Part model, mm, in its own coordinate system. Face numbers are marked on the shaded views. Round coordinates to 2 decimals unless told otherwise and drop trailing zeros. Loops run counter-clockwise (first coordinate to the right, second up) from the corner with the lowest first, then second, coordinate; pieces in that order, holes last.
from build123d import *

# Parameters (mm, degrees)
SKETCH1_W           = 40
SKETCH1_H           = 50
BOSS_EXTRUDE1_DEPTH = 5
SKETCH2_W           = 27
SKETCH2_H           = 6
SKETCH2_H_2         = 4
CUT_EXTRUDE1_DEPTH  = 6
SKETCH3_R           = 3.025
CUT_EXTRUDE2_DEPTH  = 6
LPATTERN1_COUNT     = 2
LPATTERN1_PITCH     = 12
LPATTERN1_COL_COUNT = 2
LPATTERN1_COL_PITCH = 12
FILLET1_R           = 4
FILLET2_R           = 0.5


with BuildPart() as part:
    # Sketch1 → Boss-Extrude1 (new body)
    with BuildSketch(Plane(origin=(0, 0, 0), x_dir=(1, 0, 0), z_dir=(0, 1, 0))):
        Rectangle(SKETCH1_W, SKETCH1_H)
    extrude(amount=BOSS_EXTRUDE1_DEPTH)

    # Sketch2 → Cut-Extrude1 (cut, through all)
    with BuildSketch(Plane(origin=(0, 5, 0), x_dir=(1, 0, 0), z_dir=(0, 1, 0))):
        with Locations((0, 18)):
            Rectangle(SKETCH2_W, SKETCH2_H)
        with Locations((0, 8.5)):
            Rectangle(SKETCH2_W, SKETCH2_H)
        Rectangle(SKETCH2_W, SKETCH2_H_2)
    extrude(amount=-CUT_EXTRUDE1_DEPTH, mode=Mode.SUBTRACT)

    # Sketch3 → Cut-Extrude2 (cut, through all)
    with BuildSketch(Plane(origin=(0, 5, 0), x_dir=(1, 0, 0), z_dir=(0, 1, 0))):
        with Locations((0, -10)):
            Circle(SKETCH3_R)
    cut_extrude2 = extrude(amount=-CUT_EXTRUDE2_DEPTH, mode=Mode.SUBTRACT)

    # LPattern1: Cut-Extrude2 ×2
    with Locations(*[(i * LPATTERN1_PITCH, 0, 0) for i in range(1, LPATTERN1_COUNT)]):
        add(cut_extrude2, mode=Mode.SUBTRACT)

    # LPattern1 col: Cut-Extrude2 ×2
    with Locations(*[(-i * LPATTERN1_COL_PITCH, 0, 0) for i in range(1, LPATTERN1_COL_COUNT)]):
        add(cut_extrude2, mode=Mode.SUBTRACT)

    # Fillet1
    fillet1_edges = [part.edges().sort_by_distance(p)[0] for p in [
        (20, 2.5, 25),
        (-20, 2.5, 25),
        (-20, 2.5, -25),
        (20, 2.5, -25),
    ]]
    fillet(fillet1_edges, radius=FILLET1_R)

    # Fillet2
    fillet2_edges = [part.edges().sort_by_distance(p)[0] for p in [
        (13.5, 2.5, -21),
        (13.5, 2.5, -15),
        (-13.5, 2.5, -15),
        (-13.5, 2.5, -21),
        (13.5, 2.5, -11.5),
        (13.5, 2.5, -5.5),
        (-13.5, 2.5, -5.5),
        (-13.5, 2.5, -11.5),
        (13.5, 2.5, -2),
        (13.5, 2.5, 2),
        (-13.5, 2.5, 2),
        (-13.5, 2.5, -2),
    ]]
    fillet(fillet2_edges, radius=FILLET2_R)


solid = part.part
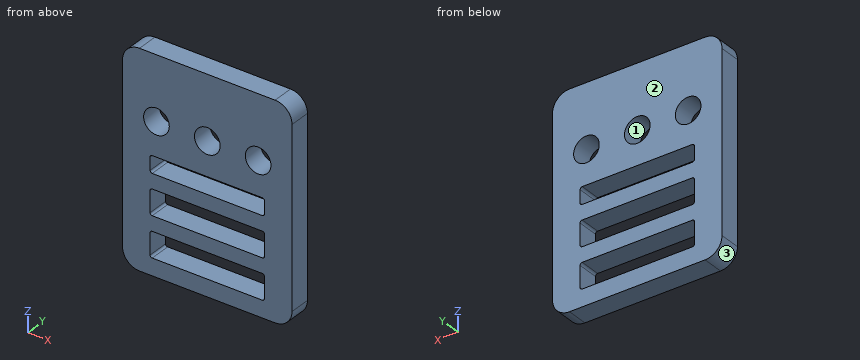
1) Slice it at A-A, the plane x = 7.5. Give the cut face in (y, z), then the cut area to 3 significant figures.
Values:
outline: (0, -25) - (5, -25) - (5, -21) - (0, -21) - close; (0, -15) - (5, -15) - (5, -11.5) - (0, -11.5) - close; (0, -5.5) - (5, -5.5) - (5, -2) - (0, -2) - close; (0, 2) - (5, 2) - (5, 25) - (0, 25) - close
area: 170 mm2
2) Slice it at B-B, the plane z = 10. Give the cut face in (x, y) (3 decimals), then the cut area to 3 significant figures.
Values:
outline: (-20, 0) - (-15.025, 0) - (-15.025, 5) - (-20, 5) - close; (-8.975, 0) - (-3.025, 0) - (-3.025, 5) - (-8.975, 5) - close; (3.025, 0) - (8.975, 0) - (8.975, 5) - (3.025, 5) - close; (15.025, 0) - (20, 0) - (20, 5) - (15.025, 5) - close
area: 109 mm2
3) Drop a flat-ended pin along its axis: pin 1 Ø3.5 at (x, z) = (12, 10) entering from -Y. Give the stop position or say it passes through.
Values:
pin 1: passes through
4) Wall check: line 1 along Z through (x, y) = (0, 1.6) (3 decimals); line 2 along X through (y, z) = (1.95, 10) (3 decimals); line 3 along Z through (x, y) = (-4, 0.3). Give the ranges that are in metal, low to high.
Values:
line 1: z = -25 to -21, -15 to -11.5, -5.5 to -2, 2 to 6.975, 13.025 to 25
line 2: x = -20 to -15.025, -8.975 to -3.025, 3.025 to 8.975, 15.025 to 20
line 3: z = -25 to -21, -15 to -11.5, -5.5 to -2, 2 to 25
5) Slice it at D-D, the plane z = -18. Give the cut face in (x, y).
Values:
outline: (-20, 0) - (-13.5, 0) - (-13.5, 5) - (-20, 5) - close; (13.5, 0) - (20, 0) - (20, 5) - (13.5, 5) - close
6) Mould opens along Z. For the marked faces 1, 2 and 3 say: released by +Z, released by -Z, zero draft, split by the parting line, or undercut.
Values:
face 1: undercut
face 2: zero draft
face 3: released by -Z
7) Slice it at C-C, the plane x = 0. Give the cut face in (y, z) (3 decimals).
Values:
outline: (0, -25) - (5, -25) - (5, -21) - (0, -21) - close; (0, -15) - (5, -15) - (5, -11.5) - (0, -11.5) - close; (0, -5.5) - (5, -5.5) - (5, -2) - (0, -2) - close; (0, 2) - (5, 2) - (5, 6.975) - (0, 6.975) - close; (0, 13.025) - (5, 13.025) - (5, 25) - (0, 25) - close
